Answer from the drawing. Dimensions are ordinates in mm from the lowest x, y and z of the part. A direction names the side the tool comes from. Round coordinates to 2 decimals unless told otherwise and drop trailing zeros. Order: outer loops, then holes, each group sorted by start corner. A loop starts at its lowest first (then second) coordinate and runs counter-clockwise, first axis right, second up. Notation, with made-up numbers: (55, 0.5) -> (96, 0.5) arc R35 cw to (96, 32.5) -> close; hole circle Ø4 at (-30, -12). An arc over 180 degrees is marked (long way). Use a Markdown table: item, result. Add a question column.
1. Given pin 1 (8 mm diameter, centred on x = 1.5, z = 22.5, fed in from -Y); pin 2 (7.5 mm diameter, centred on x = 4, y = 7.5, fed in from -Z); pin 3 (4 mm diameter, centred on y = 7.5, z = 22.5, fed in from +X); pin 4 (8 mm diameter, centred on y = 3, z = 8, fed in from +X), each flat-ended and moving along its own axis, determine where each tip first touches the part or whether it passes through.
2. Section D-D, the plane z = 23 is taken. Give the vertices of the cut face in (x, y).
3. Consider L1, parallel to Z at x = 9.75, y = 7.5; L2, parallel to Y at x = 7.5, z = 22.5; L3, parallel to Z at x = 14, y = 6.75. Determine where each line is inside the solid, lowest interval first. Write a range as [from, to].
4. Section B-B, the plane x = 7.5 is taken. Give the vertices of the cut face in (y, z).
5. For the marked faces 1, 2 and 3, determine the directions among +Z, -Z, +X, -X, +Y, -Y from which every point of the face is accessible in a straight line to the end or side of a thin tool.
6. Section A-A, the plane y = 7.5 is taken. Give the vertices of the cut face in (x, z).
7. Section C-C, the plane y = 9.75 is taken. Give the vertices of the cut face in (x, z).
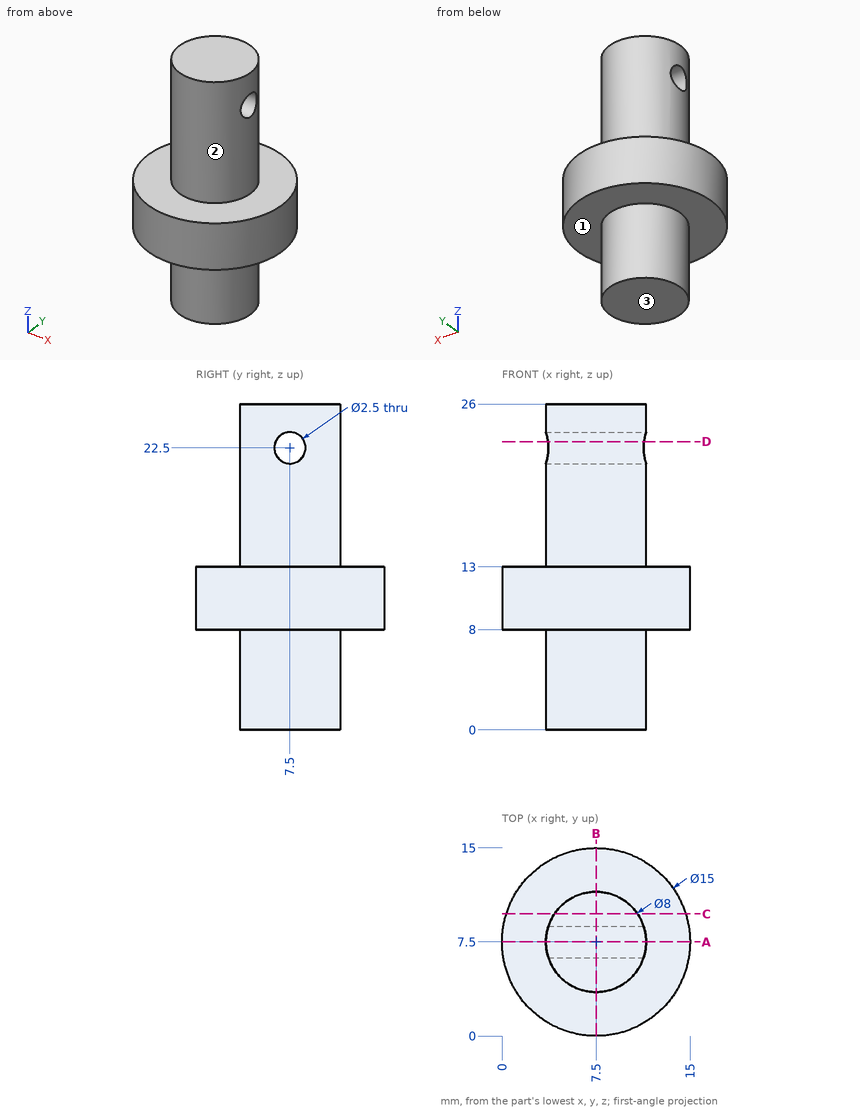
Verdict:
| question | item | result |
|---|---|---|
| 1 | pin 1 | stops at y = 4.04 |
| 1 | pin 2 | stops at z = 0 |
| 1 | pin 3 | stops at x = 11.5 |
| 1 | pin 4 | stops at x = 14.98 |
| 2 | outline | (3.67, 6.35) arc R4 ccw to (11.33, 6.35) -> close; (3.67, 8.65) -> (11.33, 8.65) arc R4 ccw to start |
| 3 | L1 | z = [0, 21.25], [23.75, 26] |
| 3 | L2 | y = [3.5, 6.25], [8.75, 11.5] |
| 3 | L3 | z = [8, 13] |
| 4 | outline | (0, 8) -> (3.5, 8) -> (3.5, 0) -> (11.5, 0) -> (11.5, 8) -> (15, 8) -> (15, 13) -> (11.5, 13) -> (11.5, 26) -> (3.5, 26) -> (3.5, 13) -> (0, 13) -> close; hole circle Ø2.5 at (7.5, 22.5) |
| 5 | face 1 | -Z |
| 5 | face 2 | +Z |
| 5 | face 3 | -Z, +X, -X, +Y, -Y |
| 6 | outline | (0, 8) -> (3.5, 8) -> (3.5, 0) -> (11.5, 0) -> (11.5, 8) -> (15, 8) -> (15, 13) -> (11.5, 13) -> (11.5, 21.25) -> (3.5, 21.25) -> (3.5, 13) -> (0, 13) -> close; (3.5, 23.75) -> (11.5, 23.75) -> (11.5, 26) -> (3.5, 26) -> close |
| 7 | outline | (0.35, 8) -> (4.19, 8) -> (4.19, 0) -> (10.81, 0) -> (10.81, 8) -> (14.65, 8) -> (14.65, 13) -> (10.81, 13) -> (10.81, 26) -> (4.19, 26) -> (4.19, 13) -> (0.35, 13) -> close |
